```python
from build123d import *

# Parameters (mm, degrees)
F0_W     = 70
F0_H     = 70
F1_DEPTH = 0.5
F2_W     = 3
F2_H     = 39
F2_R     = 1.5
F3_DEPTH = 0.501


with BuildPart() as f1:
    # F0 (on Top) → F1 (new body)
    with BuildSketch(Plane.XY):
        with Locations((-35, -35)):
            Rectangle(F0_W, F0_H)
    extrude(amount=F1_DEPTH)

    # F2 (on Top) → F3 (cut, through all)
    with BuildSketch(Plane.XY):
        with Locations((-60.5, -47.5)):
            Rectangle(F2_W, F2_H)
        with Locations((-45.5, -47.5)):
            Rectangle(F2_W, F2_H)
        with Locations((-45.5, -3)):
            Circle(F2_R)
        with Locations((-45.5, -22)):
            Circle(F2_R)
    extrude(amount=F3_DEPTH, mode=Mode.SUBTRACT)


solid = f1.part
```
Verification items for the finished model (mm, model axes). Give positions to 0.01 mm unless a question says otherwise; leave off trailing zeros. Loops run counter-clockwise (first coordinate to the right, second up) from the corner with the lowest first, then second, coordinate; pieces in that order, holes last.
1. Section check D-D, the plane z = 0.1. Enter the section's corners in (x, y).
2. Thickness scan on line 1 (X direction, y = -48, z = 0.2); line 2 (Y direction, x = -45.5, z = 0.2); line 3 (Y direction, x = -60, z = 0.1). Record the ranges inside material, lowest first.
3. Section check A-A, the plane x = -45.5. Enter the section's corners in (y, z), then the cut area to 3 significant figures.
4. Section check C-C, the plane y = -3. Enter the section's corners in (x, z).
5. Mould release check, pull along X, two halves, no side actions. Record for faces 1 (the flat face through (-35, -35, 0)), 2 (the cylindrical face through (-47, -2.93, 0.25)), 3 (the cylindrical face through (-47, -21.93, 0.25)): released by +X, released by -X, zero draft, split by the parting line, or undercut.
6. Section check B-B, the plane y = -54. Enter the section's corners in (x, z), then the cut area to 3 significant figures.
Geometry says:
1. outline: (-70, -70) - (0, -70) - (0, 0) - (-70, 0) - close; hole (-62, -67) - (-59, -67) - (-59, -28) - (-62, -28) - close; hole (-47, -67) - (-44, -67) - (-44, -28) - (-47, -28) - close; hole circle Ø3 at (-45.5, -22); hole circle Ø3 at (-45.5, -3)
2. line 1: x = -70 to -62, -59 to -47, -44 to 0
2. line 2: y = -70 to -67, -28 to -23.5, -20.5 to -4.5, -1.5 to 0
2. line 3: y = -70 to -67, -28 to 0
3. outline: (-70, 0) - (-67, 0) - (-67, 0.5) - (-70, 0.5) - close; (-28, 0) - (-23.5, 0) - (-23.5, 0.5) - (-28, 0.5) - close; (-20.5, 0) - (-4.5, 0) - (-4.5, 0.5) - (-20.5, 0.5) - close; (-1.5, 0) - (0, 0) - (0, 0.5) - (-1.5, 0.5) - close
3. area: 12.5 mm2
4. outline: (-70, 0) - (-47, 0) - (-47, 0.5) - (-70, 0.5) - close; (-44, 0) - (0, 0) - (0, 0.5) - (-44, 0.5) - close
5. face 1: zero draft
5. face 2: undercut
5. face 3: undercut
6. outline: (-70, 0) - (-62, 0) - (-62, 0.5) - (-70, 0.5) - close; (-59, 0) - (-47, 0) - (-47, 0.5) - (-59, 0.5) - close; (-44, 0) - (0, 0) - (0, 0.5) - (-44, 0.5) - close
6. area: 32.0 mm2
